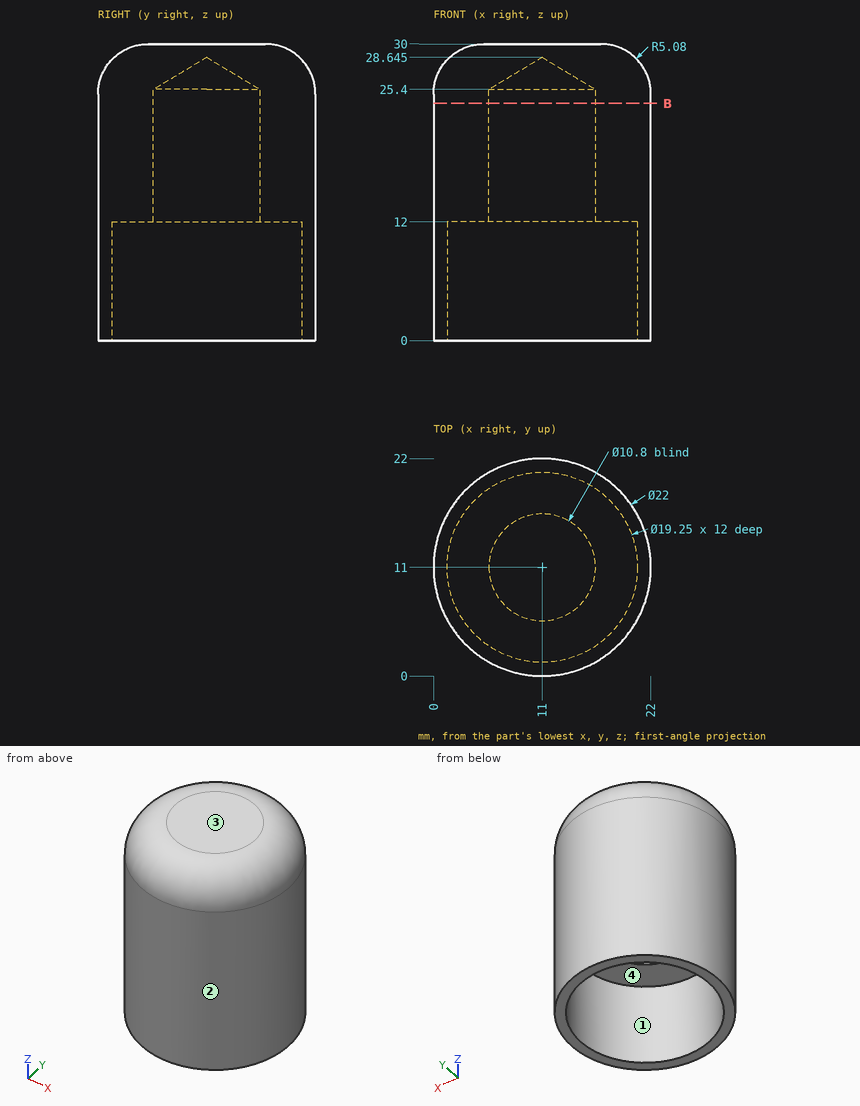
Study the drawing (mm; zero at the part's minimum x, y, z) and answer. Give positions to 0.01 mm unless a question says otherwise; leave off trailing zeros. Write each loop counter-clockwise with the first axis right and the second up, starting at its lowest first coordinate (ties: lowest second). Pieces come first, ordered by that corner, then holes.
(1) Straight lines are drawn through the part: line 1 (Y direction, x = 11, z = 5.5) (1 decimal); line 2 (Y direction, x = 11, z = 21.25); line 3 (X direction, y = 6.25, z = 2). For each, find the intervals that lie inside material, in ascending order.
Final values:
line 1: y = 0 to 1.4, 20.6 to 22
line 2: y = 0 to 5.6, 16.4 to 22
line 3: x = 1.08 to 2.63, 19.37 to 20.92
(2) The mould has two halves that part along X. Classify the marked faces 1, 2, 3 and 4: pulls with the +X half, pulls with the -X half, needs draft (parallel to the pull), parting line crosses it, or undercut.
Final values:
face 1: undercut
face 2: parting line crosses it
face 3: needs draft
face 4: undercut
(3) The part is cut by section B-B on z = 24. Write down the section's boundary in (x, y).
Final values:
outline: circle Ø22 at (11, 11); hole circle Ø10.8 at (11, 11)
(4) Flat-ended cylindrical pins translate along their axes: pin 1 Ø2 at (x, z) = (17, 25) entering from -Y; pin 2 Ø9.5 at (x, y) = (9, 11) entering from -Z; pin 3 Ø8 at (y, z) = (6, 21) entering from +X. Find the tip coordinate at first contact, or state that the pin passes through.
Final values:
pin 1: stops at y = 1.2
pin 2: stops at z = 12
pin 3: stops at x = 21.95
